Can you work these out from the model? Positions are in its coordinate system, mm. Face numbers are marked on the shaded views. A direction names the side the tool comes from. Give positions to 0.01 mm unless a question says otherwise; leave off trailing zeros. Order: outer loops, then holes, each group sorted by start corner. A loop starts at its lowest first (then second) coordinate and runs counter-clockwise, first axis right, second up. Notation, with made-up numbers: (31, -7.5) - (78, -7.5) arc R11 ccw to (78, 5.5) - close; hole circle Ø9 at (-36.75, 17). An arc over 180 degrees is marked (long way). Answer as CSV lines item,"result".
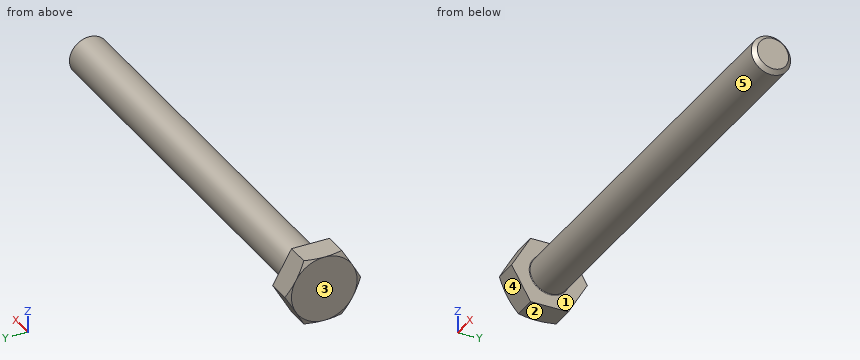
Autodesk Inventor part; units mm, degrees
ref_plane "Work Plane1" through (1.525, 0, 0) normal (0, 0, 1) x (1, 0, 0)
ref_plane "YZ Plane" through (0, 0, 0) normal (1, 0, 0) x (0, 1, 0)
ref_plane "XZ Plane" through (0, 0, 0) normal (0, 1, 0) x (-1, 0, 0)
sketch "Эскиз1" plane through (0, 0, 0) normal (0, 0, 1) x (1, 0, 0)
  line L0 (0, 3) -> (65, 3)
  line L1 (65, 3) -> (65, 0)
  line L2 (65, 0) -> (0, 0)
  line L3 (-13, 0) -> (78, 0)
  line L4 (0, -0.6) -> (0, 3.6)
  line L5 (0, 3) -> (0, 0)
  dimension "d2" = 6
  dimension "d59" = 65
revolve "Базовый элемент" add sketch "Эскиз1" angle 360 about axis through (65, 0, 0) along (-1, 0, 0)
sketch "Эскиз2" plane through (0, 0, 0) normal (-1, 0, 0) x (0, 0, 1)
  line L0 (0, 5.7735) -> (5, 2.8868)
  line L1 (5, 2.8868) -> (5, -2.8868)
  line L2 (5, -2.8868) -> (0, -5.7735)
  line L3 (0, -5.7735) -> (-5, -2.8868)
  line L4 (-5, -2.8868) -> (-5, 2.8868)
  line L5 (-5, 2.8868) -> (0, 5.7735)
  line L6 (-7, 0) -> (7, 0)
  line L7 (0, 8.0829) -> (0, -8.0829)
  point P0 (0, 0)
  point P1 (0, 0)
  dimension "d11" = 10
extrude "С головкой" add sketch "Эскиз2" along normal blind 4
sketch "Эскиз4" plane through (0, 0, 0) normal (0, 0, 1) x (1, 0, 0)
  line L0 (-3.4226, 6) -> (-4, 5)
  line L1 (-1.1, 0) -> (-0.234, 0)
  line L2 (-4.7532, 0) -> (0.5192, 0)
  line L3 (-4, 6) -> (-3.4226, 6)
  line L4 (-4, 5) -> (-4, 6)
  line L5 (0, 7.2) -> (0, -1.2)
  dimension "d65" = 10
  dimension "d67" = 30
  dimension "d68" = 12
  dimension "d69" = 4
revolve "Фаска1" cut sketch "Эскиз4" angle 360 about axis through (-1.1, 0, 0) along (1, 0, 0)
thread "Резьба"
chamfer "Фаска2" distance 0.6135 distance2 0.6136 1 edges at (65, -3, 0) measured on face at (65, -0.7485, 0.6631)
fillet "Fillet2" radius 0.1 1 edges at (0, -3, 0)
ref_plane "Work Plane1" through (1.525, 0, 0) normal (0, 0, 1) x (1, 0, 0)
equation "\"d71\" = RR"
equation "\"d11\" = SW"
equation "\"d3\" = KOH"
equation "\"d15\" = GEL"
equation "\"d6\" = -0.5 * SPD + 0.5 * GD"
equation "\"d2\" = GD"
equation "\"d59\" = NLG"
equation "\"d65\" = SW"
equation "\"d67\" = ANG1"
equation "\"d68\" = 1.2 * SW"
equation "\"d69\" = KOH"
equation "\"NLG\" = 65"
equation "\"GD\" = 6"
equation "\"BDM\" = 6"
equation "\"KOH\" = 4"
equation "\"GEL\" = 18"
equation "\"SW\" = 10"
equation "\"SW0\" = 9"
equation "\"SPD\" = NND - 1.2269 * PTC"
equation "\"SD2\" = 6"
equation "\"SD\" = 0"
equation "\"ANG1\" = 30deg"
equation "\"GAL\" = 0.61345 * PTC"
equation "\"GUL\" = 0.61345 * PTC"
equation "\"RR\" = 0.1"
equation "\"RR1\" = 0.1"
equation "\"GD1\" = THREADDIA - 1.2269 * PTC"
equation "\"THREADDIA\" = 6"
equation "\"TOA\" = 30deg"
equation "\"PTC\" = 1"
equation "\"NND\" = 6"
equation "\"E0\" = 1.155 * SW"
properties part number "Болт M6-6gx65 ГОСТ 7798-70" material "Сталь, мягкая"
1) I'm going to push a flat-ended pin straight in: P1, Ø6, axis at x = 35.5, z = 3, coming from the +Y side. Where does the tip first touch, or does it pass through?
Answer block:
P1,"y = 3"
2) I want a section at A-A on x = 54. Write out the boundary of the cut face in (y, z), plus the area to 3 significant figures.
Answer block:
outline,"circle Ø6 at (0, 0)"
area,"28.3 mm2"
3) If we mould it in two halves opening along X, with no side actions, what happens to the marked faces 1, 2 and 3? For each: +X half, -X half, draft (parallel to the pull), parting line (faces both ways), or undercut.
Answer block:
face 1,"+X half"
face 2,"draft"
face 3,"-X half"
4) Which directions (+Z, -Z, +X, -X, +Y, -Y) give clear straight access to the entire face, cutting with the end or side of a thin tool? Please do the marked faces 4 and 5.
Answer block:
face 4,"-Z, +X, -X, -Y"
face 5,"+X"
5) I need wall thicknesses on line 1 along X through (y, z) = (2.75, 4); line 2 along Y through (x, z) = (22, -0.5); line 3 along Z through (x, y) = (61.5, -2.75). Which ranges of each line are inside material? Lowest first, please. Write a range as [from, to].
Answer block:
line 1,"[-4, 0]"
line 2,"[-2.96, 2.96]"
line 3,"[-1.2, 1.2]"
